For this review, take the finished solid that the model builds, in its own axes (mm). Face numbers are marked on the shaded views. A direction names the side the tool comes from. Round coordinates to 2 decimals unless told otherwise and drop trailing zeros. Write each loop counter-clockwise with the first axis right and the second up, starting at its lowest first coordinate (ties: lowest second). Pieces come first, ordered by that corner, then holes. Notation, with made-up numbers: (-35.5, -36.75) - (-26.5, -36.75) arc R21 cw to (-26.5, -6.75) - close; hole circle Ø5 at (48.25, 24.5). An arc over 180 degrees is marked (long way). Answer in a Markdown table with one row per item. Add a question column.
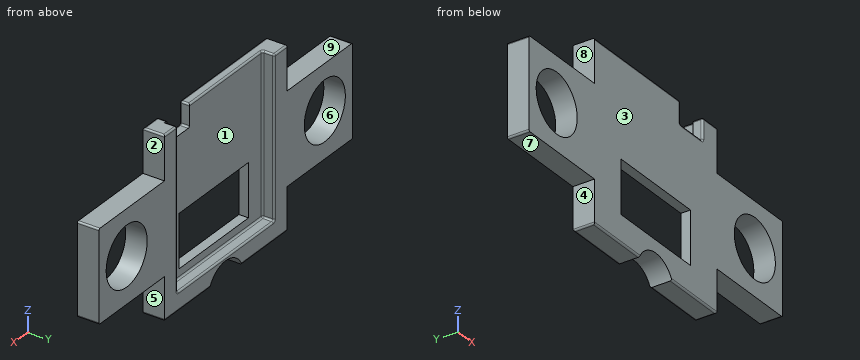
from build123d import *

# Parameters (mm, degrees)
SKETCH1_W           = 20.75
SKETCH1_H           = 20.75
SKETCH1_W_2         = 11.75
SKETCH1_H_2         = 6.2
BOSS_EXTRUDE1_DEPTH = 1.12
SKETCH2_W           = 2.15
SKETCH2_H           = 18.6
BOSS_EXTRUDE2_DEPTH = 1.4
CUT_EXTRUDE1_DEPTH  = 15.739106147
FILLET1_R           = 0.2
SKETCH5_R           = 3.475
BOSS_EXTRUDE3_DEPTH = 2.52
SKETCH6_R           = 3
CUT_EXTRUDE2_DEPTH  = 10


with BuildPart() as part:
    # Sketch1 → Boss-Extrude1 (new body)
    with BuildSketch(Plane(origin=(0, 0, 0), x_dir=(1, 0, 0), z_dir=(0, 1, 0))):
        Rectangle(SKETCH1_W, SKETCH1_H)
        with Locations((0, 4.075)):
            Rectangle(SKETCH1_W_2, SKETCH1_H_2, mode=Mode.SUBTRACT)
    extrude(amount=BOSS_EXTRUDE1_DEPTH)

    # Sketch2 → Boss-Extrude2 (add)
    with BuildSketch(Plane(origin=(0, 1.12, 0), x_dir=(1, 0, 0), z_dir=(0, 1, 0))):
        Polygon((10.375, 10.375), (-10.375, 10.375), (-10.375, 8.225), (-8.225, 8.225), (8.225, 8.225), (10.375, 8.225), align=None)
        with Locations((-9.3, -1.075)):
            Rectangle(SKETCH2_W, SKETCH2_H)
        with Locations((9.3, -1.075)):
            Rectangle(SKETCH2_W, SKETCH2_H)
    extrude(amount=BOSS_EXTRUDE2_DEPTH)

    # Sketch3 → Cut-Extrude1 (cut, through all)
    with BuildSketch(Plane(origin=(0, 1.12, 0), x_dir=(1, 0, 0), z_dir=(0, 1, 0))):
        with BuildLine():
            Line((7.925, -10.375), (4.128372784, -10.375))
            Line((4.128372784, -10.375), (4.128372784, -7.975))
            ThreePointArc((4.128372784, -7.975), (4.186951428, -7.833578644), (4.328372784, -7.775))
            Line((4.328372784, -7.775), (7.725, -7.775))
            ThreePointArc((7.725, -7.775), (7.866421356, -7.833578644), (7.925, -7.975))
            Line((7.925, -7.975), (7.925, -10.375))
        make_face()
    extrude(amount=-CUT_EXTRUDE1_DEPTH, mode=Mode.SUBTRACT)

    # Fillet1
    fillet1_edges = [part.edges().sort_by_distance(p)[0] for p in [
        (-2.048313608, 1.12, 10.375),
        (-8.225, 1.82, -8.225),
        (0, 1.12, -8.225),
        (-8.225, 2.52, 1.075),
        (-8.225, 1.82, 10.375),
        (-9.3, 2.52, 10.375),
        (0, 2.52, -8.225),
        (8.225, 2.52, 1.075),
        (0, 2.52, -10.375),
        (-8.225, 1.12, 1.075),
        (8.225, 1.82, -8.225),
        (9.3, 2.52, 10.375),
        (8.225, 1.82, 10.375),
        (-3.123313608, 0, 10.375),
        (0, 0, -10.375),
        (9.15, 0, 10.375),
        (7.925, 0, 9.175),
        (7.925, 0.56, 10.375),
        (4.128372784, 0, 9.175),
        (4.128372784, 0.56, 10.375),
        (4.186951428, 0, 7.833578644),
        (6.026686392, 0, 7.775),
        (7.866421356, 0, 7.833578644),
        (10.375, 1.26, 10.375),
        (-10.375, 1.26, -10.375),
        (10.375, 1.26, -10.375),
    ]]
    fillet(fillet1_edges, radius=FILLET1_R)

    # Sketch5 → Boss-Extrude3 (add)
    # profile 1 of 2: a face of its own
    with BuildSketch(Plane(origin=(0, 2.52, 0), x_dir=(1, 0, 0), z_dir=(0, 1, 0))):
        with BuildLine():
            Line((-10.375, 5.392486931), (-21.275499471, 5.392486931))
            ThreePointArc((-21.275499471, 5.392486931), (-21.416920828, 5.333908287), (-21.475499471, 5.192486931))
            Line((-21.475499471, 5.192486931), (-21.475499471, -5.096478262))
            ThreePointArc((-21.475499471, -5.096478262), (-21.416920828, -5.237899618), (-21.275499471, -5.296478262))
            Line((-21.275499471, -5.296478262), (-10.375, -5.296478262))
            Line((-10.375, -5.296478262), (-10.375, 5.392486931))
        make_face()
        with Locations(Location((-16.77, 0, 0), (0, 0, 270))):
            Circle(SKETCH5_R, mode=Mode.SUBTRACT)
    # profile 2 of 2: a face of its own
    with BuildSketch(Plane(origin=(0, 2.52, 0), x_dir=(1, 0, 0), z_dir=(0, 1, 0))):
        with BuildLine():
            Line((10.375, 5.392486931), (21.275499471, 5.392486931))
            ThreePointArc((21.275499471, 5.392486931), (21.416920828, 5.333908287), (21.475499471, 5.192486931))
            Line((21.475499471, 5.192486931), (21.475499471, -5.096478262))
            ThreePointArc((21.475499471, -5.096478262), (21.416920828, -5.237899618), (21.275499471, -5.296478262))
            Line((21.275499471, -5.296478262), (10.375, -5.296478262))
            Line((10.375, -5.296478262), (10.375, 5.392486931))
        make_face()
        with Locations(Location((16.77, 0, 0), (0, 0, 270))):
            Circle(SKETCH5_R, mode=Mode.SUBTRACT)
    extrude(amount=-BOSS_EXTRUDE3_DEPTH)

    # Sketch6 → Cut-Extrude2 (cut)
    with BuildSketch(Plane(origin=(0, 2.52, 0), x_dir=(1, 0, 0), z_dir=(0, 1, 0))):
        with Locations((0, 11.63)):
            Circle(SKETCH6_R)
    extrude(amount=-CUT_EXTRUDE2_DEPTH, mode=Mode.SUBTRACT)


solid = part.part
Q1. To check wall thickness, follow probe 1 along X at (y, z) = (0.7, 0) (1 decimal); probe 2 along X at (y, z) = (1.85, 0) (1 decimal); probe 3 along Z at (x, y) = (-17, 0.65). State the ranges of each line that lie inside material, in increasing order.
Q2. Tool access review of the marked faces 1, 2, 3, 4 and 5: name each direction out of +Z, -Z, +X, -X, +Y, -Y from which nothing blocks a thin tool from reaching the whole face with its end or side.
Q3. Insertion check: pin 1 Ø1 at (x, y) = (-12, 1.5) entering from -Z; pin 2 Ø0.9 at (x, y) = (-2, 0.5) entering from -Z; pin 3 Ø0.8 at (y, z) = (1.5, 7) entering from -X (3 decimals). Each pin has a flat end and moves straight along its axis. Give the tip position at first contact, or say it passes through.
Q4. Add section C-C on x = 0.5. State the section outline as (y, z) points (3 decimals).
Q5. Add section B-B on x = 16.77. State the section outline as (y, z) points (3 decimals).
Q6. Add section A-A on z = 0. Count the separate pieces of the cut face and the enclosed holes in it, then the cut area to 3 significant figures.
Q7. Add section D-D on x = -18.5. State the section outline as (y, z) points, then the cut area to 3 significant figures.
Q8. Draft analysis for pull direction Z (two halves, no side actions). For the marked faces 6, 7, 8 and 9, state which applies: released by +Z, released by -Z, zero draft, split by the parting line, or undercut.
Answer sheet:
| question | item | result |
|---|---|---|
| 1 | probe 1 | x = -21.5 to -20.2, -13.3 to 13.3, 20.2 to 21.5 |
| 1 | probe 2 | x = -21.5 to -20.2, -13.3 to -8.2, 8.2 to 13.3, 20.2 to 21.5 |
| 1 | probe 3 | z = -5.39 to -3.47, 3.47 to 5.3 |
| 2 | face 1 | +Z, +Y |
| 2 | face 2 | +Z, +X, +Y, -Y |
| 2 | face 3 | +Z, -Z, +X, -X, -Y |
| 2 | face 4 | -Z, -X, +Y, -Y |
| 2 | face 5 | -Z, +X, +Y, -Y |
| 3 | pin 1 | stops at z = -5.39 |
| 3 | pin 2 | stops at z = -9.9 |
| 3 | pin 3 | stops at x = -10.375 |
| 4 | outline | (0, -8.672) - (2.52, -8.672) - (2.52, -8.425) arc R0.2 ccw to (2.32, -8.225) - (1.32, -8.225) arc R0.2 cw to (1.12, -8.025) - (1.12, -7.175) - (0, -7.175) - close; (0, -0.975) - (1.12, -0.975) - (1.12, 10.175) arc R0.2 ccw to (0.92, 10.375) - (0.2, 10.375) arc R0.2 ccw to (0, 10.175) - close |
| 5 | outline | (0, -5.392) - (2.52, -5.392) - (2.52, -3.475) - (0, -3.475) - close; (0, 3.475) - (2.52, 3.475) - (2.52, 5.296) - (0, 5.296) - close |
| 6 | separate pieces | 3 |
| 6 | enclosed holes | 0 |
| 6 | area | 50.2 mm² |
| 7 | outline | (0, -5.39) - (2.52, -5.39) - (2.52, -3.01) - (0, -3.01) - close; (0, 3.01) - (2.52, 3.01) - (2.52, 5.3) - (0, 5.3) - close |
| 7 | area | 11.7 mm² |
| 8 | face 6 | undercut |
| 8 | face 7 | released by -Z |
| 8 | face 8 | zero draft |
| 8 | face 9 | released by +Z |
